Read the model definition and answer for the solid it produces. Units are mm, in the model's axes. A direction names the side the tool comes from. Coordinates: 2 decimals unless noted, no trailing zeros. Write each loop counter-clockwise with the first axis right and the second up, starting at its lowest first coordinate (ties: lowest second). Pieces come first, ordered by that corner, then holes.
(1) Given pin 1 (2 mm diameter, centred on x = -4, y = 94.5, fed in from -Z); pin 2 (1.5 mm diameter, centred on x = 0.5, y = 69.5, fed in from +Z); pin 3 (2 mm diameter, centred on y = 24, z = -1.5, fed in from -X), each flat-ended and moving along its own axis, determine where each tip first touches the part or whether it passes through.
(2) Which of the six approach directions +Z, -Z, +X, -X, +Y, -Y give full straight-line access (tool end or side, diameter ignored) to faces 1 (the flat face through (-7.332, 3.465, 4.301)), 2 (the flat face through (-7.39, 3.46, -4.2)), 3 (the flat face through (6, 14, -4))?
(3) Determine the mould class of faces 4 (the cylindrical face through (-7.542, 6.565, 4.286)), 5 (the flat face through (7.332, 3.465, -4.301)), 6 (the cylindrical face through (2, 125, 0)), 7 (the flat face through (-1, 8, 0)) for opening direction X: pulls with the +X half, pulls with the -X half, needs draft (parallel to the pull), parting line crosses it, or undercut.
(4) Straight lines are drawn through the part: line 1 along X through (y, z) = (3, 0); line 2 along X through (y, z) = (125.35, 0); line 3 along Y through (x, z) = (5, 0.75). For each, find the intervals that lie inside material, in ascending order.
(5) The part is cut by section A-A, the plane y = 74.5. Determine the outline of the cut face in (x, z).
(6) The part is cut by section B-B, the plane y = -27. Determine the outline of the cut face in (x, z).
```python
from build123d import *

# Parameters (mm, degrees)
ESQUISSE2_R             = 4
ENL_V_MAT_EXTRU_1_DEPTH = 8
ENL_V_START             = -9
ENL_V_MAT_EXTRU_2_DEPTH = 9
ESQUISSE4_R             = 15
ENL_V_MAT_EXTRU_3_DEPTH = 7
CONG_1_R                = 1
ESQUISSE5_R             = 0.5
BOSS_EXTRU_1_DEPTH      = 80


with BuildPart() as part:
    # Esquisse1 → Révolution1 (revolve)
    with BuildSketch(Plane.XY, mode=Mode.PRIVATE) as r_volution1_sk:
        Polygon((4, 127), (4, 27), (7, 27), (7, 14), (9.5, 14), (9.5, 0), (0, 0), (0, 121), (2, 123), (2, 127), align=None)
    revolve(r_volution1_sk.sketch.rotate(Axis((0, 0, 0), (0, 1, 0)), 90), axis=Axis((0, 0, 0), (0, 1, 0)))

    # Esquisse2 → Enlèv. mat.-Extru.1 (cut)
    with BuildSketch(Plane.XZ):
        with Locations(Location((0, 0, 0), (0, 0, 270))):
            Circle(ESQUISSE2_R)
    extrude(amount=-ENL_V_MAT_EXTRU_1_DEPTH, mode=Mode.SUBTRACT)

    # Esquisse3 → Enlèv. mat.-Extru.2 (cut)
    with BuildSketch(Plane(origin=(0, 27, 0), x_dir=(1, 0, 0), z_dir=(0, 1, 0)).offset(ENL_V_START)):
        with BuildLine():
            Line((6, -3.605551275), (6, 3.605551275))
            ThreePointArc((6, 3.605551275), (7, 0), (6, -3.605551275))
        make_face()
        with BuildLine():
            Line((-6, -3.605551275), (-6, 3.605551275))
            ThreePointArc((-6, 3.605551275), (-7, 0), (-6, -3.605551275))
        make_face()
    extrude(amount=ENL_V_MAT_EXTRU_2_DEPTH, mode=Mode.SUBTRACT)

    # Esquisse4 → Enlèv. mat.-Extru.3 (cut)
    with BuildSketch(Plane.XZ):
        Circle(ESQUISSE4_R)
        Polygon((9.814954576, 0), (4.907477288, 8.5), (-4.907477288, 8.5), (-9.814954576, 0), (-4.907477288, -8.5), (4.907477288, -8.5), align=None, mode=Mode.SUBTRACT)
    extrude(amount=-ENL_V_MAT_EXTRU_3_DEPTH, mode=Mode.SUBTRACT)

    # Congé1
    cong_1_edges = [part.edges().sort_by_distance(p)[0] for p in [
        (0, 127, 4),
        (-3.446820352, 27, -6.092571663),
        (0, 27, 7),
        (0, 0, -8.5),
        (-4.75, 0, -8.227241336),
        (-7.361215932, 0, -4.25),
        (-9.5, 0, 0),
        (-7.361215932, 0, 4.25),
        (-4.75, 0, 8.227241336),
        (0, 0, 8.5),
        (4.75, 0, 8.227241336),
        (7.361215932, 0, 4.25),
        (9.5, 0, 0),
        (7.361215932, 0, -4.25),
        (4.75, 0, -8.227241336),
        (0, 0, 4),
        (0, 7, 8.5),
        (7.361215932, 7, 4.25),
        (7.361215932, 7, -4.25),
        (0, 7, -8.5),
        (-7.361215932, 7, -4.25),
        (-7.361215932, 7, 4.25),
    ]]
    fillet(cong_1_edges, radius=CONG_1_R - 0.0001)  # a hair under: the kernel refuses the full size

    # Esquisse5 → Boss.-Extru.1 (add)
    with BuildSketch(Plane.XZ.offset(-8)):
        with Locations(Location((0, 0, 0), (0, 0, 270))):
            Circle(ESQUISSE5_R)
    extrude(amount=BOSS_EXTRU_1_DEPTH)


solid = part.part
```
Computed:
1. pin 1: stops at z = -2.65
1. pin 2: stops at z = 4
1. pin 3: stops at x = -6
2. face 1: +Z, -X, -Y
2. face 2: -Z, -X, -Y
2. face 3: +Y
3. face 4: pulls with the -X half
3. face 5: pulls with the +X half
3. face 6: undercut
3. face 7: undercut
4. line 1: x = -9.5 to -4, -0.5 to 0.5, 4 to 9.5
4. line 2: x = -4 to -2, 2 to 4
4. line 3: y = 0 to 27
5. outline: circle Ø8 at (0, 0)
6. outline: circle Ø1 at (0, 0)
